Geometry: final body of the model. Coordinates: model frame, mm. A direction names the side the tool comes from. Give positions to 0.01 mm unless a question says otherwise; leave off trailing zeros. Order: outer loops, then holes, each group sorted by start corner. A loop starts at its lowest first (then second) coordinate and runs counter-clockwise, first axis right, second up. Notation, with made-up numbers: (53.5, 85) - (91.5, 85) arc R9 cw to (91.5, 89) - close; hole circle Ø11 at (18.25, 29.5). An arc over 180 degrees is marked (long way). One line per item, written item: value.
```python
from build123d import *

# Parameters (mm, degrees)
SKETCH1_W           = 20.955
SKETCH1_H           = 14.859
BOSS_EXTRUDE1_DEPTH = 7.62
CUT_EXTRUDE1_DEPTH  = 15.859
SKETCH3_R           = 2.8575
CUT_EXTRUDE2_DEPTH  = 4.683
SKETCH4_R           = 0.9271
CUT_EXTRUDE3_DEPTH  = 3.81


with BuildPart() as part:
    # Sketch1 → Boss-Extrude1 (new body)
    with BuildSketch(Plane(origin=(0, 0, 0), x_dir=(1, 0, 0), z_dir=(0, 1, 0))):
        with Locations((10.4775, 7.4295)):
            Rectangle(SKETCH1_W, SKETCH1_H)
    extrude(amount=BOSS_EXTRUDE1_DEPTH)

    # Sketch2 → Cut-Extrude1 (cut, through all)
    with BuildSketch(Plane.XY):
        Polygon((5.6515, 7.62), (1.143, 7.62), (3.39725, 5.36575), align=None)
        Polygon((14.1605, 7.62), (6.7945, 7.62), (10.4775, 3.937), align=None)
        Polygon((19.812, 7.62), (15.3035, 7.62), (17.55775, 5.36575), align=None)
    extrude(amount=-CUT_EXTRUDE1_DEPTH, mode=Mode.SUBTRACT)

    # Sketch3 → Cut-Extrude2 (cut, through all)
    with BuildSketch(Plane(origin=(0, 3.937, 0), x_dir=(1, 0, 0), z_dir=(0, 1, 0))):
        with Locations((10.4775, 7.4295)):
            Circle(SKETCH3_R)
    extrude(amount=CUT_EXTRUDE2_DEPTH, mode=Mode.SUBTRACT)

    # Sketch4 → Cut-Extrude3 (cut)
    with BuildSketch(Plane.XZ):
        with Locations((4.0386, -3.7846)):
            Circle(SKETCH4_R)
        with Locations((4.0386, -11.0744)):
            Circle(SKETCH4_R)
        with Locations((10.4775, -7.4295)):
            Circle(SKETCH4_R)
        with Locations((16.9164, -11.0744)):
            Circle(SKETCH4_R)
        with Locations((16.9164, -3.7846)):
            Circle(SKETCH4_R)
    extrude(amount=-CUT_EXTRUDE3_DEPTH, mode=Mode.SUBTRACT)


solid = part.part
```
1) Mould query, pull axis Z, two halves, no side actions, for faces 5 (the face through (4.51, 6.48, -7.33)), 6 (the face through (17, 3.81, -11)), 7 (the face through (10, 3, 0)). Classes: released by +Z, released by -Z, zero draft, split by the parting line, or undercut.
Answers below:
face 5: zero draft
face 6: undercut
face 7: released by +Z
2) Set-up query: faces 1 (the face through (13.334, 5.028, -7.367)), 2 (the face through (6, 7.62, -8)), 3 (the face through (2.254, 6.509, -7.325)), 4 (the face through (10.91, 1.88, -8.25)). Return all of +Z, -Z, +X, -X, +Y, -Y with unobstructed straight access to the full face (end or side cutting, diameter ignored); none if empty.
Answers below:
face 1: +Y
face 2: +Z, -Z, +X, -X, +Y
face 3: +Z, -Z, +Y
face 4: -Y
3) Section D-D, the plane y = 0.5. Return loops of the section in (x, z) (1 decimal).
Answers below:
outline: (0, -14.9) - (21, -14.9) - (21, 0) - (0, 0) - close; hole circle Ø1.9 at (4, -11.1); hole circle Ø1.9 at (4, -3.8); hole circle Ø1.9 at (10.5, -7.4); hole circle Ø1.9 at (16.9, -11.1); hole circle Ø1.9 at (16.9, -3.8)
4) Material intervals for line 1 along X through (y, z) = (5.75, -12) (1 decimal); line 2 along X through (y, z) = (3.25, -4.5) (3 decimals); line 3 along Z through (x, y) = (17.75, 0.5), sorted ascending.
Answers below:
line 1: 0 to 3, 3.8 to 8.7, 12.3 to 17.2, 17.9 to 21
line 2: 0 to 3.449, 4.628 to 16.327, 17.506 to 20.955
line 3: -14.86 to -11.48, -10.67 to -4.19, -3.38 to 0
5) Section A-A, the plane z = -12.5. Return loops of the section in (x, y) (1 decimal), then the cut area to 3 significant figures.
Answers below:
outline: (0, 0) - (21, 0) - (21, 7.6) - (19.8, 7.6) - (17.6, 5.4) - (15.3, 7.6) - (14.2, 7.6) - (10.5, 3.9) - (6.8, 7.6) - (5.7, 7.6) - (3.4, 5.4) - (1.1, 7.6) - (0, 7.6) - close
area: 136 mm^2
6) Section C-C, the plane x = 12.25. Return loops of the section in (y, z).
Answers below:
outline: (0, -14.86) - (5.71, -14.86) - (5.71, -9.67) - (3.94, -9.67) - (3.94, -5.19) - (5.71, -5.19) - (5.71, 0) - (0, 0) - close
7) Section B-B, the plane y = 5.75. Return loops of the section in (x, z) (1 decimal).
Answers below:
outline: (0, -14.9) - (3, -14.9) - (3, 0) - (0, 0) - close; (3.8, -14.9) - (8.7, -14.9) - (8.7, -9.6) arc R2.9 cw to (8.7, -5.2) - (8.7, 0) - (3.8, 0) - close; (12.3, -14.9) - (17.2, -14.9) - (17.2, 0) - (12.3, 0) - (12.3, -5.2) arc R2.9 cw to (12.3, -9.6) - close; (17.9, -14.9) - (21, -14.9) - (21, 0) - (17.9, 0) - close
8) First-contact query: pin 1 (2 mm diameter, centred on x = 4, z = -11.5, fed in from -Y); pin 2 (1.1 mm diameter, centred on x = 16.92, z = -3.78, fed in from +Y); pin 3 (1.5 mm diameter, centred on x = 11, z = -5, fed in from +Y); pin 4 (1.5 mm diameter, centred on x = 9.5, z = -5, fed in from +Y). Flat tips, straight axial feed; report the tip coordinate or a pass-through.
Answers below:
pin 1: y = 0
pin 2: y = 6.55
pin 3: y = 5.2
pin 4: y = 5.66
